Geometry: final body of the model. Coordinates: model frame, mm. Face numbers are marked on the shaded views. Round coordinates to 2 decimals unless told otherwise and drop trailing zeros. Write each loop counter-clockwise with the first axis right and the second up, starting at its lowest first coordinate (ties: lowest second). Pieces come first, ordered by that corner, then holes. Notation, with made-up numbers: M -10.75,33.25 L 13.25,33.25 A30 cw 13.25,55.25 Z; hole C 81.25,65.5 d9. An arc over 180 degrees is marked long. Use one line per item in the form item = value. Start each with the question number.
Item 1: Ray query, probe 1 along Y at (x, z) = (0, 103); probe 2 along X at (y, z) = (-35, 22); probe 3 along Y at (x, z) = (-31, 151.5). Return the intervals inside material, ascending.
Item 2: Section query A-A (z = 22.5). Return loops of the section in (x, y).
Item 3: Pull-direction query (Z, two-part tool) for the marked faces 1, 2 and 3; classes: pulls with the +Z half, pulls with the -Z half, needs draft (parallel to the pull), parting line crosses it, or undercut.
Item 4: Pin query (flat end, axial travel): pin 1 Ø3 at (x, y) = (-33, 46) entering from +Z; pin 2 Ø5 at (x, z) = (-2.5, -56.5) entering from +Y; pin 3 Ø2 at (y, z) = (-4.5, 43) entering from -X; pin 4 Ø12 at (y, z) = (45, -29.5) entering from +X. Return the tip coordinate at first contact, or that it passes through.
Item 5: Section query B-B (z = -68). Return loops of the section in (x, y), and give its area (3 significant figures).
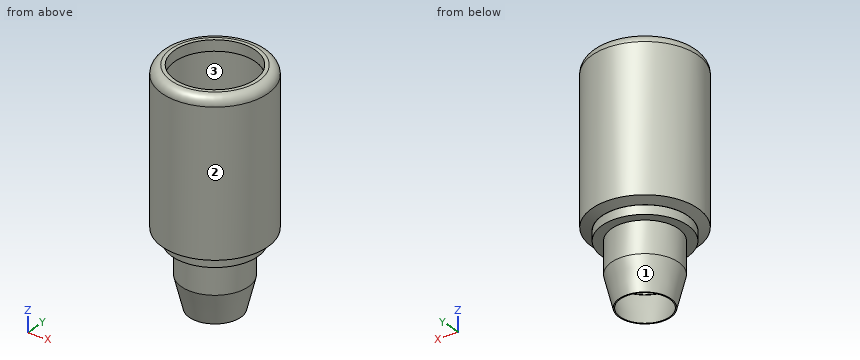
Autodesk Inventor part; units mm, degrees
ref_plane "YZ Plane" through (0, 0, 0) normal (1, 0, 0) x (0, 1, 0)
ref_plane "XZ Plane" through (0, 0, 0) normal (0, 1, 0) x (-1, 0, 0)
ref_plane "XY Plane" through (0, 0, 0) normal (0, 0, 1) x (1, 0, 0)
sketch "Эскиз1" plane through (0, 0, 0) normal (0, 0, 1) x (1, 0, 0)
  circle A0 centre (0, 0) radius 59
  dimension "d0" = 118
extrude "Выдавливание1" add sketch "Эскиз1" along normal blind 150
extrude "Выдавливание2" add sketch "Эскиз1" against normal blind 4 draft -70
sketch "Эскиз2" plane through (0, 0, -4) normal (0, 0, -1) x (-1, 0, 0)
  circle A0 centre (0, 0) radius 47.803848
extrude "Выдавливание3" add sketch "Эскиз2" along normal blind 10
sketch "Эскиз3" plane through (0, 0, -14) normal (0, 0, -1) x (-1, 0, 0)
  circle A0 centre (0, 0) radius 37.5
  circle A1 centre (0, 0) radius 36.5
  dimension "d7" = 75
  dimension "d20" = 73
extrude "Выдавливание4" add sketch "Эскиз3" along normal blind 35 contours A0 | A1
sketch "Эскиз4" plane through (0, 0, -49) normal (0, 0, -1) x (-1, 0, 0)
  point P0 (0, 0)
sketch "Эскиз5" plane through (0, 0, -49) normal (0, 0, -1) x (-1, 0, 0)
  circle A0 centre (0, 0) radius 37.5
  circle A1 centre (0, 0) radius 35
  dimension "d16" = 70
sketch "Эскиз5 outline for Выдавливание5" plane through (0, 0, -49) normal (0, 0, -1) x (-1, 0, 0)
  circle A0 centre (0, 0) radius 37.5
extrude "Выдавливание5" add sketch "Эскиз5 outline for Выдавливание5" along normal blind 35 draft -14
sketch "Эскиз6" plane through (0, 0, 150) normal (0, 0, 1) x (1, 0, 0)
  circle A0 centre (0, 0) radius 59
  circle A1 centre (0, 0) radius 45
  dimension "d12" = 90
extrude "Выдавливание6" add sketch "Эскиз6" along normal blind 20
fillet "Сопряжение1" radius 10 1 edges at (-59, 0, 170)
sketch "Эскиз7" plane through (0, 0, -84) normal (0, 0, -1) x (-1, 0, 0)
  circle A0 centre (0, 0) radius 28.77352
  circle A1 centre (0, 0) radius 27.5
  dimension "d17" = 55
extrude "Выдавливание7" cut sketch "Эскиз7" against normal blind 35 draft 15 contours A1
sketch "Эскиз8" plane through (0, 0, -49) normal (0, 0, -1) x (-1, 0, 0)
  circle A0 centre (0, 0) radius 36.5
  dimension "d21" = 73
extrude "Выдавливание8" cut sketch "Эскиз8" against normal blind 35
sketch "Эскиз9" plane through (0, 0, -14) normal (0, 0, -1) x (-1, 0, 0)
  circle A0 centre (0, 0) radius 36.5
  dimension "d24" = 73
extrude "Выдавливание9" cut sketch "Эскиз9" against normal blind 10
sketch "Эскиз10" plane through (0, 0, -4) normal (0, 0, -1) x (-1, 0, 0)
  circle A0 centre (0, 0) radius 36.5
  dimension "d27" = 73
extrude "Выдавливание10" cut sketch "Эскиз10" against normal blind 4 draft 78
sketch "Эскиз11" plane through (0, 0, 0) normal (0, 0, -1) x (-1, 0, 0)
  circle A0 centre (0, 0) radius 58
  dimension "d30" = 116
extrude "Выдавливание11" cut sketch "Эскиз11" against normal blind 158
properties part number "Колибри-Шаблон"
Working result:
q1.probe_1 = -59 to -58, 58 to 59
q1.probe_2 = -47.5 to -46.25, 46.25 to 47.5
q1.probe_3 = -50.2 to -49.02, 49.02 to 50.2
q2.outline = C 0,0 d118; hole C 0,0 d116
q3.face_1 = pulls with the -Z half
q3.face_2 = needs draft
q3.face_3 = undercut
q4.pin_1 = 167.91
q4.pin_2 = 36.19
q4.pin_3 = -58.9
q4.pin_4 = through
q5.outline = C 0,0 d65.53; hole C 0,0 d63.57
q5.area = 198 mm²
